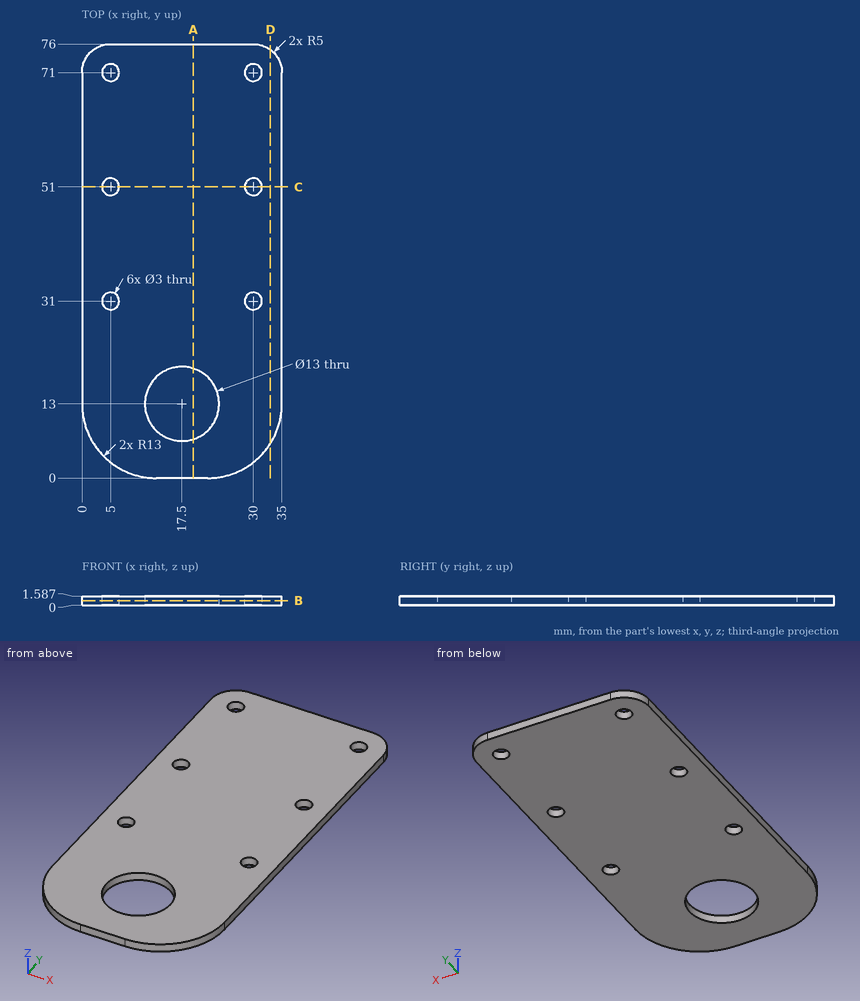
Study the drawing (mm; zero at the part's minimum x, y, z) and answer. Give positions to 0.01 mm unless a question says otherwise; leave off trailing zeros. Write each loop counter-clockwise with the first axis right and the second up, starting at its lowest first coordinate (ties: lowest second). Pieces come first, ordered by that corner, then holes. Notation, with made-up numbers: (-14, 75) - (31, 75) arc R23 cw to (31, 100) - close; hole circle Ø4 at (61, -29). An arc over 180 degrees is marked (long way). Use CSV: the item, a comma, the result in double quotes. Start each with the question number.
(1) Find section D-D (x = 33). Give the vertices of the cut face in (y, z).
(2) Consider line 1 along X through (y, z) = (71, 1.2); line 2 along Y through (x, z) = (30, 0.35) (1 decimal); line 3 along Y through (x, z) = (17.5, 0.5). Determine where each line is inside the solid, lowest interval first.
(3) Given P1, Ø21, axis at x = 17.5, y = 13, coming from the -Z side; P2, Ø1.8, axis at x = 30, y = 31, coming from the +Z side, each flat-ended and moving along its own axis, determine where each tip first touches the part or whether it passes through.
(4) Find section B-B (z = 0.8). Give the vertices of the cut face in (x, y), plus the area to 3 significant figures.
(5) Find section C-C (y = 51). Give the vertices of the cut face in (x, z).
(6) Find section A-A (x = 19.5). Give the vertices of the cut face in (y, z) (1 decimal).
Findings below:
1,outline,"(6.07, 0) - (75, 0) - (75, 1.59) - (6.07, 1.59) - close"
2,line 1,"0 to 3.5, 6.5 to 28.5, 31.5 to 35"
2,line 2,"2.8 to 29.5, 32.5 to 49.5, 52.5 to 69.5, 72.5 to 76"
2,line 3,"0 to 6.5, 19.5 to 76"
3,P1,"z = 0"
3,P2,"through"
4,outline,"(0, 13) arc R13 ccw to (13, 0) - (22, 0) arc R13 ccw to (35, 13) - (35, 71) arc R5 ccw to (30, 76) - (5, 76) arc R5 ccw to (0, 71) - close; hole circle Ø3 at (5, 31); hole circle Ø3 at (5, 51); hole circle Ø3 at (5, 71); hole circle Ø13 at (17.5, 13); hole circle Ø3 at (30, 31); hole circle Ø3 at (30, 51); hole circle Ø3 at (30, 71)"
4,area,"2,400 mm2"
5,outline,"(0, 0) - (3.5, 0) - (3.5, 1.59) - (0, 1.59) - close; (6.5, 0) - (28.5, 0) - (28.5, 1.59) - (6.5, 1.59) - close; (31.5, 0) - (35, 0) - (35, 1.59) - (31.5, 1.59) - close"
6,outline,"(0, 0) - (6.8, 0) - (6.8, 1.6) - (0, 1.6) - close; (19.2, 0) - (76, 0) - (76, 1.6) - (19.2, 1.6) - close"
